Build history of the part. All positions in model axes, mm. A direction names the side the tool comes from. Round coordinates to 2 decimals unless told otherwise and drop trailing zeros. Write each loop counter-clockwise with the first axis right and the second up, starting at its lowest first coordinate (ties: lowest second). Pieces come first, ordered by that corner, then holes.
1) Flat gauge pins, fed straight in: pin 1 (1 mm diameter, centred on x = 4.5, y = 13, fed in from +Z); pin 2 (3 mm diameter, centred on x = -13, z = 3, fed in from -Y); pin 3 (8 mm diameter, centred on y = -3, z = 7, fed in from -X). Where does each tip first touch, or does it go through?
2) Saw through at C-C (y = -13). Write the cut outline in (x, z), plus the area to 3 significant figures.
3) Wall check: probe 1 along X at (y, z) = (14, 5); probe 2 along Z at (x, y) = (15, 12.75); probe 3 along X at (y, z) = (13, 6.5). Give the ranges that are in metal, low to high.
4) Which spindle directions (+Z, -Z, +X, -X, +Y, -Y) get a long thin tool onto all of the face, cutting with end or side? Do faces 4 (the flat face through (0, -20, 5)), 5 (the flat face through (13, 10, 5)), 6 (the flat face through (-10, -5, 5)). Say none if no direction does.
5) Saw through at A-A (z = 5). Write the cut outline in (x, y), plus the area to 3 significant figures.
6) Saw through at B-B (x = 15). Write the cut outline in (y, z).
7) Pull direction Z, two halves, no side cores. Call faces 1 (the cylindrical face through (-0.9, -17, 14.4)), 2 (the cylindrical face through (13.885, 15.07, 6.216)), 3 (the flat face through (0, 5, 10)): +Z half, -Z half, draft (parallel to the pull), parting line (faces both ways), or undercut.
8) Saw through at D-D (y = 11.5). Write the cut outline in (x, z).
from build123d import *

# Parameters (mm, degrees)
SKETCH_1_W          = 10
SKETCH_1_H          = 10
SKETCH_1_W_2        = 20
SKETCH_1_H_2        = 40
EXTRUDE_5_DEPTH     = 10
SKETCH_7_R          = 4.1
EXTRUDE_6_DEPTH     = 9
SKETCH_8_R          = 1.65
CUT_EXTRUDE_1_DEPTH = 10


with BuildPart() as part:
    # Эскиз1 → Бобышка-Вытянуть5 (new body)
    with BuildSketch(Plane.XY):
        with Locations((-15, 15)):
            Rectangle(SKETCH_1_W, SKETCH_1_H)
        Rectangle(SKETCH_1_W_2, SKETCH_1_H_2)
        with Locations((15, 15)):
            Rectangle(SKETCH_1_W, SKETCH_1_H)
    extrude(amount=EXTRUDE_5_DEPTH)

    # Эскиз7 → Бобышка-Вытянуть6 (add)
    with BuildSketch(Plane.XY.offset(10)):
        with Locations((0, -13)):
            Circle(SKETCH_7_R)
    extrude(amount=EXTRUDE_6_DEPTH)

    # Эскиз8 → Вырез-Вытянуть1 (cut)
    with BuildSketch(Plane(origin=(0, 20, 0), x_dir=(1, 0, 0), z_dir=(0, 1, 0))):
        with Locations(Location((-15, -5, 0), (0, 0, 270))):
            Circle(SKETCH_8_R)
        with Locations(Location((15, -5, 0), (0, 0, 90))):
            Circle(SKETCH_8_R)
    extrude(amount=-CUT_EXTRUDE_1_DEPTH, mode=Mode.SUBTRACT)


solid = part.part
Evaluation:
1. pin 1: stops at z = 10
1. pin 2: stops at y = 10
1. pin 3: stops at x = -10
2. outline: (-10, 0) - (10, 0) - (10, 10) - (4.1, 10) - (4.1, 19) - (-4.1, 19) - (-4.1, 10) - (-10, 10) - close
2. area: 274 mm2
3. probe 1: x = -20 to -16.65, -13.35 to 13.35, 16.65 to 20
3. probe 2: z = 0 to 3.35, 6.65 to 10
3. probe 3: x = -20 to -15.69, -14.31 to 14.31, 15.69 to 20
4. face 4: +Z, -Z, +X, -X, -Y
4. face 5: +Z, -Z, +X, -Y
4. face 6: +Z, -Z, -X, -Y
5. outline: (-20, 10) - (-16.65, 10) - (-16.65, 20) - (-20, 20) - close; (-13.35, 10) - (-10, 10) - (-10, -20) - (10, -20) - (10, 10) - (13.35, 10) - (13.35, 20) - (-13.35, 20) - close; (16.65, 10) - (20, 10) - (20, 20) - (16.65, 20) - close
5. area: 934 mm2
6. outline: (10, 0) - (20, 0) - (20, 3.35) - (10, 3.35) - close; (10, 6.65) - (20, 6.65) - (20, 10) - (10, 10) - close
7. face 1: draft
7. face 2: undercut
7. face 3: +Z half
8. outline: (-20, 0) - (20, 0) - (20, 10) - (-20, 10) - close; hole circle Ø3.3 at (-15, 5); hole circle Ø3.3 at (15, 5)
